The model under review builds one solid part; all positions refer to its coordinate system, in mm. Face numbers are marked on the shaded views. Round coordinates to 2 decimals unless told otherwise and drop trailing zeros. Loops run counter-clockwise (first coordinate to the right, second up) from the corner with the lowest first, then second, coordinate; pieces in that order, holes last. Notation, with made-up numbers: (-21.5, 76) -> (-15.5, 76) arc R10 ccw to (-15.5, 80) -> close; hole circle Ø4 at (-28, 34.25). An arc over 180 degrees is marked (long way). Use a Markdown table: item, result. Add a question column.
1) Wall thickness on probe 1 along Z at (x, y) = (22.45, -7.75); probe 2 along X at (y, z) = (-12.5, 24); probe 3 along Z at (x, y) = (0, -5.25): over which ranges is each line inside the solid? List them lowest first.
2) Mouldability with a two-part tool opening along X and no side actions: class the marked faces 1, 2 and 3 as released by +X, released by -X, zero draft, split by the parting line, or undercut.
3) Consider section D-D on x = 0. Give the boundary of the cut face in (y, z).
4) Consider section A-A on z = 0. Give the boundary of the cut face in (x, y), plus the area to 3 significant figures.
5) Consider section C-C on z = 22.45. Give the boundary of the cut face in (x, y), plus the area to 3 significant figures.
6) Insertion check: pin 1 (1.9 mm diameter, centred on y = -6.5, z = -1.5, fed in from -X); pin 2 (4 mm diameter, centred on x = 22.45, z = 22.45, fed in from -Y); pin 3 (5 mm diameter, centred on y = -7.5, z = 2, fed in from -X); pin 4 (1.9 mm diameter, centred on y = -8, z = -1, fed in from +X). Each pin has a flat end and moves straight along its axis. Give the tip position at first contact, or say it passes through.
7) Consider section B-B on x = 22.45. Give the boundary of the cut face in (y, z), plus the area to 3 significant figures.
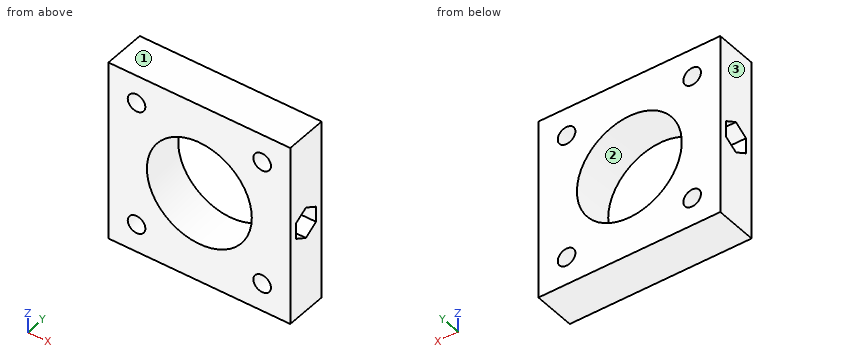
Solid Edge part; units mm, degrees
sketch "Sketch1" plane through (0, 0, 0) normal (0, -1, 0) x (1, 0, 0)
  line L0 (32.5, -32.5) -> (32.5, 32.5)
  line L1 (32.5, 32.5) -> (-32.5, 32.5)
  line L2 (-32.5, 32.5) -> (-32.5, -32.5)
  line L3 (-32.5, -32.5) -> (32.5, -32.5)
  circle A0 centre (0, 0) radius 18.75
extrude "Protrusion1" add sketch "Sketch1" along normal blind 15
sketch "Sketch2" plane through (-32.5, -7.5, 0) normal (-1, 0, 0) x (0, -1, 0)
  line L0 (4.85, 2.8001) -> (0, 5.6003)
  line L1 (0, 5.6003) -> (-4.85, 2.8001)
  line L2 (-4.85, 2.8001) -> (-4.85, -2.8001)
  line L3 (-4.85, -2.8001) -> (0, -5.6003)
  line L4 (0, -5.6003) -> (4.85, -2.8001)
  line L5 (4.85, -2.8001) -> (4.85, 2.8001)
extrude "ExtrudedCutout_2" cut sketch "Sketch2" against normal blind 8.1
sketch "Sketch3" plane through (32.5, -7.5, 0) normal (1, 0, 0) x (0, 1, 0)
  line L0 (-4.85, -2.8001) -> (0, -5.6003)
  line L1 (0, -5.6003) -> (4.85, -2.8001)
  line L2 (4.85, -2.8001) -> (4.85, 2.8001)
  line L3 (4.85, 2.8001) -> (0, 5.6003)
  line L4 (0, 5.6003) -> (-4.85, 2.8001)
  line L5 (-4.85, 2.8001) -> (-4.85, -2.8001)
extrude "ExtrudedCutout_3" cut sketch "Sketch3" against normal blind 8.1
sketch "Sketch4" plane through (-24.4, -7.5, 0) normal (-1, 0, 0) x (0, -0.866, -0.5)
  circle A0 centre (0, 0) radius 3.15
extrude "ExtrudedCutout_4" cut sketch "Sketch4" against normal blind 0.5
sketch "Sketch5" plane through (24.4, -7.5, 0) normal (1, 0, 0) x (0, 0.866, -0.5)
  circle A0 centre (0, 0) radius 3.15
extrude "ExtrudedCutout_5" cut sketch "Sketch5" against normal blind 0.5
sketch "Sketch6" plane through (0, 0, 0) normal (0, 1, 0) x (-1, 0, 0)
  circle A0 centre (-22.45, 22.45) radius 3.15
  circle A1 centre (22.45, 22.45) radius 3.15
  circle A2 centre (22.45, -22.45) radius 3.15
  circle A3 centre (-22.45, -22.45) radius 3.15
extrude "Cutout1" cut sketch "Sketch6" against normal up to next
Result set:
| question | item | result |
|---|---|---|
| 1 | probe 1 | -32.5 to -25.6, -19.3 to 19.3, 25.6 to 32.5 |
| 1 | probe 2 | -32.5 to -25.19, -19.71 to 19.71, 25.19 to 32.5 |
| 1 | probe 3 | -32.5 to -18.75, 18.75 to 32.5 |
| 2 | face 1 | zero draft |
| 2 | face 2 | undercut |
| 2 | face 3 | released by -X |
| 3 | outline | (-15, -32.5) -> (0, -32.5) -> (0, -18.75) -> (-15, -18.75) -> close; (-15, 18.75) -> (0, 18.75) -> (0, 32.5) -> (-15, 32.5) -> close |
| 4 | outline | (-32.5, -15) -> (-18.75, -15) -> (-18.75, 0) -> (-32.5, 0) -> (-32.5, -2.65) -> (-24.4, -2.65) -> (-24.4, -4.35) -> (-23.9, -4.35) -> (-23.9, -10.65) -> (-24.4, -10.65) -> (-24.4, -12.35) -> (-32.5, -12.35) -> close; (18.75, -15) -> (32.5, -15) -> (32.5, -12.35) -> (24.4, -12.35) -> (24.4, -10.65) -> (23.9, -10.65) -> (23.9, -4.35) -> (24.4, -4.35) -> (24.4, -2.65) -> (32.5, -2.65) -> (32.5, 0) -> (18.75, 0) -> close |
| 4 | area | 249 mm2 |
| 5 | outline | (-32.5, -15) -> (-25.6, -15) -> (-25.6, 0) -> (-32.5, 0) -> close; (-19.3, -15) -> (19.3, -15) -> (19.3, 0) -> (-19.3, 0) -> close; (25.6, -15) -> (32.5, -15) -> (32.5, 0) -> (25.6, 0) -> close |
| 5 | area | 786 mm2 |
| 6 | pin 1 | x = -23.9 |
| 6 | pin 2 | through |
| 6 | pin 3 | x = -24.4 |
| 6 | pin 4 | x = 23.9 |
| 7 | outline | (-15, -32.5) -> (0, -32.5) -> (0, -25.6) -> (-15, -25.6) -> close; (-15, -19.3) -> (0, -19.3) -> (0, 19.3) -> (-15, 19.3) -> close; (-15, 25.6) -> (0, 25.6) -> (0, 32.5) -> (-15, 32.5) -> close |
| 7 | area | 786 mm2 |
